For this review, take the finished solid that the model builds, in its own axes (mm). A direction names the side the tool comes from. Coordinates: 2 decimals unless noted, no trailing zeros. Write each loop counter-clockwise with the first axis right and the second up, starting at its lowest first coordinate (ties: lowest second). Pieces come first, ordered by that corner, then holes.
1) We need section A-A on x = 0. Write out the cut boundary in (y, z), then the cut area to 3 significant figures.
2) Insertion check: P1, Ø1.5, axis at x = 23.5, z = 10, coming from the -Y side; P2, Ø4, axis at x = 22.5, y = -23.5, coming from the +Z side; P3, Ø6.5, axis at x = -3, y = -17.5, coming from the +Z side. Each pin has a flat end and moves straight along its axis. Give the tip position at first contact, or say it passes through.
3) We need section C-C on z = 11.5. Write out the cut boundary in (x, y), then the cut area to 3 significant figures.
4) To check wall thickness, follow line 1 along X through (y, z) = (-12.5, 12); line 2 along X through (y, z) = (0, 6.75); line 3 along Y through (x, z) = (0, 8.75). State the ranges of each line that lie inside material, in increasing order.
5) We need section D-D on y = 22. Write out the cut boundary in (x, z).
6) For faces 1 (the face through (8, 12, 0)), 2 (the face through (33.31, -21.64, 10.12)), 3 (the face through (-35.56, 0, 11)), list the 3-axis set-ups (+Z, -Z, +X, -X, +Y, -Y) from which the entire face can be reached by the end or side of a thin tool; tool diameter is ignored.
7) Mouldability with a two-part tool opening along X and no side actions: class faces 4 (the face through (-32, 0, 10.16)), 5 (the face through (-1, -25.4, 6)) as pulls with the +X half, pulls with the -X half, needs draft (parallel to the pull), parting line crosses it, or undercut.
8) We need section B-B on y = 0. Write out the cut boundary in (x, z), then the cut area to 3 significant figures.
from build123d import *

# Parameters (mm, degrees)
F0_W     = 76.2
F0_H     = 50.8
F0_R     = 12.7
F1_DEPTH = 12.7
F2_W     = 6.35
F2_H     = 50.8
F3_DEPTH = 2.54
F5_DEPTH = 7.62


with BuildPart() as f1:
    # F0 (on Top) → F1 (new body)
    with BuildSketch(Plane.XY):
        Rectangle(F0_W, F0_H)
        Circle(F0_R, mode=Mode.SUBTRACT)
    extrude(amount=F1_DEPTH)

    # F2 (on face) → F3 (cut)
    with BuildSketch(Plane.XY.offset(12.7)):
        with Locations((-32.385, 0)):
            Rectangle(F2_W, F2_H)
        with BuildLine():
            Line((6.35, 25.4), (-6.35, 25.4))
            Line((-6.35, 25.4), (-6.35, 10.9985226281))
            ThreePointArc((-6.35, 10.9985226281), (0, 12.7), (6.35, 10.9985226281))
            Line((6.35, 10.9985226281), (6.35, 25.4))
        make_face()
        with BuildLine():
            Line((-6.35, -10.9985226281), (-6.35, -25.4))
            Line((-6.35, -25.4), (6.35, -25.4))
            Line((6.35, -25.4), (6.35, -10.9985226281))
            ThreePointArc((6.35, -10.9985226281), (0, -12.7), (-6.35, -10.9985226281))
        make_face()
    extrude(amount=-F3_DEPTH, mode=Mode.SUBTRACT)

    # F4 (on face) → F5 (cut)
    with BuildSketch(Plane.XZ.offset(25.4)):
        Polygon((31.8187926716, 12.7), (19.1187926716, 12.7), (16.1858533041, 7.62), (34.7517320391, 7.62), align=None)
    extrude(amount=-F5_DEPTH, mode=Mode.SUBTRACT)


solid = f1.part
Result:
1. outline: (-25.4, 0) - (-12.7, 0) - (-12.7, 10.16) - (-25.4, 10.16) - close; (12.7, 0) - (25.4, 0) - (25.4, 10.16) - (12.7, 10.16) - close
1. area: 258 mm2
2. P1: stops at y = -17.78
2. P2: stops at z = 7.62
2. P3: stops at z = 10.16
3. outline: (-38.1, -25.4) - (-35.56, -25.4) - (-35.56, 25.4) - (-38.1, 25.4) - close; (-29.21, -25.4) - (-6.35, -25.4) - (-6.35, -11) arc R12.7 cw to (-6.35, 11) - (-6.35, 25.4) - (-29.21, 25.4) - close; (6.35, -25.4) - (18.43, -25.4) - (18.43, -17.78) - (32.51, -17.78) - (32.51, -25.4) - (38.1, -25.4) - (38.1, 25.4) - (6.35, 25.4) - (6.35, 11) arc R12.7 cw to (6.35, -11) - close
3. area: 2,600 mm2
4. line 1: x = -38.1 to -35.56, -29.21 to -6.35, 6.35 to 38.1
4. line 2: x = -38.1 to -12.7, 12.7 to 38.1
4. line 3: y = -25.4 to -12.7, 12.7 to 25.4
5. outline: (-38.1, 0) - (38.1, 0) - (38.1, 12.7) - (6.35, 12.7) - (6.35, 10.16) - (-6.35, 10.16) - (-6.35, 12.7) - (-29.21, 12.7) - (-29.21, 10.16) - (-35.56, 10.16) - (-35.56, 12.7) - (-38.1, 12.7) - close
6. face 1: -Z, +X, -X, +Y, -Y
6. face 2: -Y
6. face 3: +Z, +Y, -Y
7. face 4: undercut
7. face 5: needs draft
8. outline: (-38.1, 0) - (-12.7, 0) - (-12.7, 12.7) - (-29.21, 12.7) - (-29.21, 10.16) - (-35.56, 10.16) - (-35.56, 12.7) - (-38.1, 12.7) - close; (12.7, 0) - (38.1, 0) - (38.1, 12.7) - (12.7, 12.7) - close
8. area: 629 mm2
